Design review of the part shown in the three views and the two pictorial views. Dimensions are in mm from the part's minimum x, y and z. A direction names the side the tool comes from. Round coordinates to 2 decimals unless told otherwise and drop trailing zeros. Use one line per item in the form item = value.
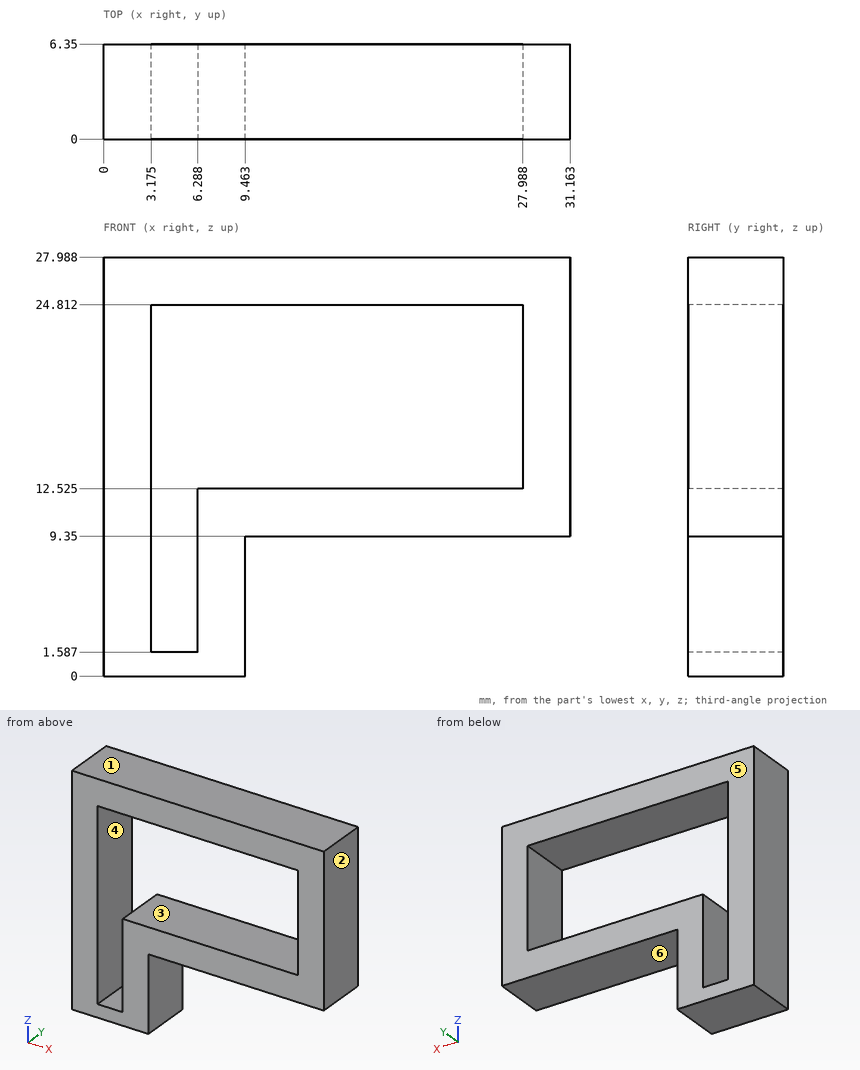
Q1. To check wall thickness, follow line 1 along X through (y, z) = (5.25, 3.25) (1 decimal); line 2 along X through (y, z) = (3.75, 13.5) (1 decimal); line 3 along Z through (x, y) = (8, 5.75) (1 decimal). State the ranges of each line that lie inside material, in increasing order. Write a range as from..to.
Calculated:
line_1 = 0..3.2, 6.3..9.5
line_2 = 0..3.2, 28..31.2
line_3 = 0..12.5, 24.8..28
Q2. Machinability: for the marked faces 4, 5 and 6, which of the approach directions +Z, -Z, +X, -X, +Y, -Y give a long, thin tool a straight path to every point of the face, cutting with its end or side? Answer none if there is none.
Calculated:
face_4 = +Y, -Y
face_5 = +Z, -Z, +X, -X, +Y
face_6 = -Z, +X, +Y, -Y
Q3. Draft analysis for pull direction Z (two halves, no side actions). For the marked faces 1, 2 and 3, state which applies: released by +Z, released by -Z, zero draft, split by the parting line, or undercut.
Calculated:
face_1 = released by +Z
face_2 = zero draft
face_3 = undercut
Q4. For P1, Ø4, axis at x = 10, z = 24.5, coming from the -Y side; P2, Ø3, axis at x = 23, y = 2, coming from the -Z side, all flat-tipped, find the tip position at first contact; note any pin that passes through.
Calculated:
P1 = 0
P2 = 9.35
